```python
from build123d import *

# Parameters (mm, degrees)
SKETCH1_W           = 127
SKETCH1_H           = 72.39
BOSS_EXTRUDE1_DEPTH = 76.2
SKETCH2_W           = 124.5616
SKETCH2_H           = 69.9516
CUT_EXTRUDE1_DEPTH  = 73.914
SKETCH4_W           = 81.28
SKETCH4_H           = 38.1
CUT_EXTRUDE2_DEPTH  = 1.2192
SKETCH5_R           = 17.145
CUT_EXTRUDE3_DEPTH  = 2.286


with BuildPart() as part:
    # Sketch1 → Boss-Extrude1 (new body)
    with BuildSketch(Plane(origin=(0, 0, 0), x_dir=(1, 0, 0), z_dir=(0, 1, 0))):
        Rectangle(SKETCH1_W, SKETCH1_H)
    extrude(amount=BOSS_EXTRUDE1_DEPTH)

    # Sketch2 → Cut-Extrude1 (cut)
    with BuildSketch(Plane(origin=(0, 76.2, 0), x_dir=(1, 0, 0), z_dir=(0, 1, 0))):
        Rectangle(SKETCH2_W, SKETCH2_H)
    extrude(amount=-CUT_EXTRUDE1_DEPTH, mode=Mode.SUBTRACT)

    # Sketch4 → Cut-Extrude2 (cut)
    with BuildSketch(Plane.XY.offset(36.195)):
        with Locations((-1.27, 57.15)):
            Rectangle(SKETCH4_W, SKETCH4_H)
    extrude(amount=-CUT_EXTRUDE2_DEPTH, mode=Mode.SUBTRACT)

    # Sketch5 → Cut-Extrude3 (cut)
    with BuildSketch(Plane.XZ):
        with Locations((-33.528, -5.207)):
            Circle(SKETCH5_R)
        with Locations((33.528, -5.207)):
            Circle(SKETCH5_R)
    extrude(amount=-CUT_EXTRUDE3_DEPTH, mode=Mode.SUBTRACT)


solid = part.part
```
Input: part model. Units: mm. Frame: model coordinates. A direction names the side the tool comes from. Round coordinates to 2 decimals unless told otherwise and drop trailing zeros. Loops run counter-clockwise (first coordinate to the right, second up) from the corner with the lowest first, then second, coordinate; pieces in that order, holes last. Notation, with made-up numbers: (69.25, -31.5) -> (101.25, -31.5) arc R9 cw to (101.25, -24.5) -> close; hole circle Ø7 at (29, 30.25). An arc over 180 degrees is marked (long way). Use one line per item in the form item = value. Start each with the question number.
Item 1: Mould query, pull axis Z, two halves, no side actions, for faces 3 (the face through (-1, 2.286, 0)), 4 (the face through (63.5, 38, 1)), 5 (the face through (-50.656, 1.127, -4.453)), 6 (the face through (-1, 29, 36.195)). Classes: pulls with the +Z half, pulls with the -Z half, needs draft (parallel to the pull), parting line crosses it, or undercut.
Item 2: Section query B-B on x = 38. Return the cut outline in (y, z) (1 decimal).
Item 3: Section query C-C on z = 9.5. Return the cut outline in (x, y), then the cut area to 3 significant figures.
Item 4: Material intervals for L1, parallel to X at y = 68.5, z = 26; L2, parallel to Z at x = 37, y = 34.5 (3 decimals); L3, parallel to Y at x = -53, z = 33, sorted ascending. Write a range as from..to.
Item 5: Set-up query: faces 1 (the face through (-63.5, 38, 1)), 2 (the face through (-1, 32, 34.976)). Return all of +Z, -Z, +X, -X, +Y, -Y with unobstructed straight access to the full face (end or side cutting, diameter ignored); none if empty.
Item 6: Section query A-A on y = 63.5. Return the cut outline in (x, z) (3 decimals).
Item 7: Section query D-D on y = 20. Return the cut outline in (x, z) (3 decimals).
Item 8: Contact query for flat-ended pins moving along their axis: pin 1 Ø1 at (x, z) = (-16, 35.5) entering from +Y; pin 2 Ø8 at (x, z) = (47, -28) entering from +Y; pin 3 Ø6 at (x, y) = (22.5, 58.5) entering from +Z. Output: stop coordinate, or through.
Ans:
q1.face_3 = undercut
q1.face_4 = needs draft
q1.face_5 = undercut
q1.face_6 = pulls with the +Z half
q2.outline = (0, -36.2) -> (76.2, -36.2) -> (76.2, -35) -> (2.3, -35) -> (2.3, -21.8) -> (0, -21.8) -> close; (0, 11.3) -> (2.3, 11.3) -> (2.3, 35) -> (38.1, 35) -> (38.1, 36.2) -> (0, 36.2) -> close
q3.outline = (-63.5, 0) -> (-42.34, 0) -> (-42.34, 2.29) -> (-62.28, 2.29) -> (-62.28, 76.2) -> (-63.5, 76.2) -> close; (-24.72, 0) -> (24.72, 0) -> (24.72, 2.29) -> (-24.72, 2.29) -> close; (42.34, 0) -> (63.5, 0) -> (63.5, 76.2) -> (62.28, 76.2) -> (62.28, 2.29) -> (42.34, 2.29) -> close
q3.area = 390 mm^2
q4.L1 = -63.5..-62.28, 62.28..63.5
q4.L2 = -36.195..-34.976, 34.976..36.195
q4.L3 = 0..2.29
q5.face_1 = +Z, -Z, -X, +Y, -Y
q5.face_2 = +Y
q6.outline = (-63.5, -36.195) -> (63.5, -36.195) -> (63.5, 36.195) -> (39.37, 36.195) -> (39.37, 34.976) -> (62.281, 34.976) -> (62.281, -34.976) -> (-62.281, -34.976) -> (-62.281, 34.976) -> (-41.91, 34.976) -> (-41.91, 36.195) -> (-63.5, 36.195) -> close
q7.outline = (-63.5, -36.195) -> (63.5, -36.195) -> (63.5, 36.195) -> (-63.5, 36.195) -> close; hole (-62.281, -34.976) -> (62.281, -34.976) -> (62.281, 34.976) -> (-62.281, 34.976) -> close
q8.pin_1 = 38.1
q8.pin_2 = 2.29
q8.pin_3 = -34.98
